Geometry: final body of the model. Coordinates: model frame, mm. Round coordinates to 2 decimals unless told otherwise and drop trailing zeros. Loops run counter-clockwise (first coordinate to the right, second up) from the corner with the lowest first, then second, coordinate; pieces in that order, holes last. Notation, with made-up numbers: M 83.25,66.5 L 87.25,66.5 A20 ccw 87.25,91.5 Z; hole C 46,63.5 d3. An arc over 180 degrees is marked long. Answer as a JSON object with one key per item and string values.
from build123d import *

# Parameters (mm, degrees)
SKETCH2_W           = 75.5
SKETCH2_H           = 30.5
BOSS_EXTRUDE2_DEPTH = 120.5
SKETCH4_W           = 75
SKETCH4_H           = 30
CUT_EXTRUDE1_DEPTH  = 120
SKETCH5_W           = 75
SKETCH5_H           = 120
CUT_EXTRUDE2_DEPTH  = 30
SKETCH6_W           = 120
SKETCH6_H           = 30
CUT_EXTRUDE3_DEPTH  = 75


with BuildPart() as part:
    # Sketch2 → Boss-Extrude2 (new body)
    with BuildSketch(Plane.XY):
        with Locations((37.75, 15.25)):
            Rectangle(SKETCH2_W, SKETCH2_H)
    extrude(amount=-BOSS_EXTRUDE2_DEPTH)

    # Sketch4 → Cut-Extrude1 (cut)
    with BuildSketch(Plane.XY):
        with Locations((37.75, 15.25)):
            Rectangle(SKETCH4_W, SKETCH4_H)
    extrude(amount=-CUT_EXTRUDE1_DEPTH, mode=Mode.SUBTRACT)

    # Sketch5 → Cut-Extrude2 (cut)
    with BuildSketch(Plane(origin=(0, 30.5, 0), x_dir=(1, 0, 0), z_dir=(0, 1, 0))):
        with Locations((37.75, 60.25)):
            Rectangle(SKETCH5_W, SKETCH5_H)
    extrude(amount=-CUT_EXTRUDE2_DEPTH, mode=Mode.SUBTRACT)

    # Sketch6 → Cut-Extrude3 (cut)
    with BuildSketch(Plane(origin=(75.5, 0, 0), x_dir=(0, 0, -1), z_dir=(1, 0, 0))):
        with Locations((60.25, 15.25)):
            Rectangle(SKETCH6_W, SKETCH6_H)
    extrude(amount=-CUT_EXTRUDE3_DEPTH, mode=Mode.SUBTRACT)


solid = part.part
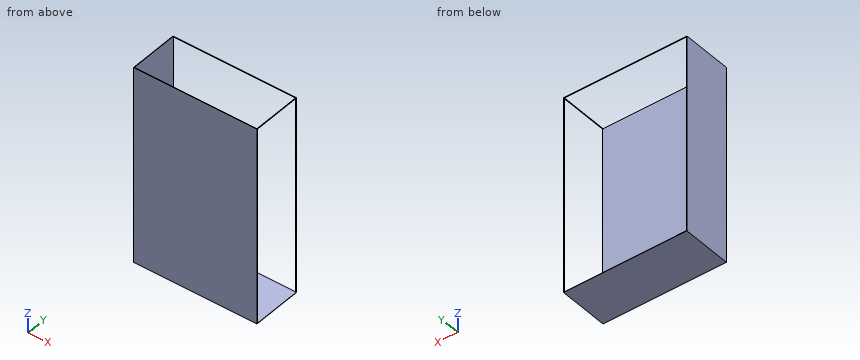
1) Ray query, line 1 (X direction, y = 28, z = -72); line 2 (Z direction, x = 69, y = 17). Return the intervals inside material, ascending.
Results:
{"line 1": "0 to 0.25", "line 2": "-120.5 to -120.25"}
2) Section query B-B (y = 16). Return the cut outline in (x, z).
Results:
{"outline": "M 0,-120.5 L 75.5,-120.5 L 75.5,-120.25 L 0.25,-120.25 L 0.25,0 L 0,0 Z; M 75.25,-0.25 L 75.5,-0.25 L 75.5,0 L 75.25,0 Z"}
3) Pin query (flat end, axial travel): P1, Ø2, axis at y = 13, z = -74.5, coming from the -X side; P2, Ø2, axis at x = 51.5, y = 11.5, coming from the +Z side. Return the tip coordinate at first contact, or that it passes through.
Results:
{"P1": "x = 0", "P2": "z = -120.25"}
4) Section query A-A (z = -69). Return the cut outline in (x, y).
Results:
{"outline": "M 0,0 L 75.5,0 L 75.5,0.25 L 0.25,0.25 L 0.25,30.5 L 0,30.5 Z; M 75.25,30.25 L 75.5,30.25 L 75.5,30.5 L 75.25,30.5 Z"}
